Could you check a few things on this model? Use its own coordinates, in mm. A direction names the side the tool comes from. Round coordinates to 2 decimals unless told otherwise and drop trailing zeros. Loops run counter-clockwise (first coordinate to the right, second up) from the corner with the lowest first, then second, coordinate; pieces in that order, holes last. Notation, with made-up numbers: (-19.5, 88) -> (5.5, 88) arc R22 ccw to (5.5, 116) -> close; hole circle Ø8 at (49, 22.25). An arc over 180 degrees is marked (long way). Put each result on its own line as item: value. Start each with the question number.
1. Which directions (+Z, -Z, +X, -X, +Y, -Y) give clear straight access to the entire face, cutting with the end or side of a thin tool? Please do faces 1 (the flat face through (-30, 47, 14.237)), 2 (the flat face through (-16, 59, 17.767)), 3 (the cylindrical face through (-70.46, 71.27, 13.74)), 4 (the flat face through (-64, 12, 17.707)).
2. Imagine slicing it at C-C, the plane x = -95. Please give me the cut outline in (y, z).
3. Imagine slicing it at A-A, the plane z = 15.5. Please give me the cut outline in (x, y), and give its area (3 significant figures).
4. If we mould it in two halves opening along Y, with no side actions, what happens to faces 5 (the cylindrical face through (-3.177, 3.795, 13.744)), 6 (the conical face through (-18.69, 54.37, 13.46)), 7 (the flat face through (-74.272, 72, 14)), 8 (the cylindrical face through (-20.557, 52.705, 13.744))? For each: pulls with the +Y half, pulls with the -Y half, needs draft (parallel to the pull), parting line crosses it, or undercut.
5. Imagine slicing it at B-B, the plane y = -19. Please give me the cut outline in (x, z), and give its area (3 significant figures).
6. I'm going to push flat-ended pins straight in: P1, Ø2, axis at y = 24, z = 15.5, coming from the +X side; P2, Ø12, axis at x = -22.5, y = 30.5, coming from the +Z side; P3, Ø20, axis at x = -74.27, y = 0, coming from the +Z side; P4, Ø1.7, axis at x = 6.5, z = 16, coming from the -Y side. Where does each tip first touch, or does it pass through?
7. I need wall thicknesses on line 1 (Z direction, x = -11.5, y = 10.5); line 2 (Y direction, x = -69.5, z = 18.25); line 3 (Y direction, x = -32, z = 14.8). Which ranges of each line are inside material? Lowest first, please. Write a range as [from, to].
```python
from build123d import *

# Parameters (mm, degrees)
REVOLVE1_ANGLE          = 90
BOSS_EXTRUDE1_START     = -1
SKETCH2_R               = 12.5
BOSS_EXTRUDE1_DEPTH     = 1
CUT_EXTRUDE1_DEPTH      = 143.444465377
CUT_EXTRUDE1_DEPTH_BACK = 143.444465377


with BuildPart() as part:
    # Sketch1 → Revolve1 (revolve)
    with BuildSketch(Plane(origin=(0, 0, 0), x_dir=(1, 0, 0), z_dir=(0, 1, 0))):
        Polygon((-16.271625609, -17.706954757), (-19.271625609, -17.706954757), (-19.271625609, -18.706954757), (-15.861337675, -18.706954757), (-11.331165057, -14.237179487), (2.840396891, -14.237179487), (7.310172161, -18.767352105), (15.728322279, -18.767352105), (15.728322279, -17.767352105), (7.728322279, -17.767352105), (3.258547009, -13.237179487), (-11.741452991, -13.237179487), align=None)
    revolve(axis=Axis((-74.271677721, 0, 17.706954757), (0, 0, 1)), revolution_arc=REVOLVE1_ANGLE)

    # Sketch2 → Boss-Extrude1 (add)
    with BuildSketch(Plane(origin=(0, 0, 17.706954757), x_dir=(-1, 0, 0), z_dir=(0, 0, -1)).offset(BOSS_EXTRUDE1_START)):
        with BuildLine():
            Line((67.342979074, 35.326946302), (59.371742963, 52.943344025))
            ThreePointArc((59.371742963, 52.943344025), (33.582268097, 37.005103388), (20.15595474, 9.823149116))
            Line((20.15595474, 9.823149116), (39.208104561, 8.157563191))
            ThreePointArc((39.208104561, 8.157563191), (99.279307908, -25.89630152), (67.342979074, 35.326946302))
        make_face()
        with Locations((74.271677721, 0)):
            Circle(SKETCH2_R, mode=Mode.SUBTRACT)
    extrude(amount=BOSS_EXTRUDE1_DEPTH)

    # Sketch3 → Cut-Extrude1 (cut, two sides: drawn at the far end of the back side and taken through both)
    with BuildSketch(Plane(origin=(0, 0, 13.237179487), x_dir=(-1, 0, 0), z_dir=(0, 0, -1)).offset(-CUT_EXTRUDE1_DEPTH_BACK)):
        with BuildLine():
            ThreePointArc((7.421193768, 7.350328837), (3.090443615, 3.801635214), (-0.54921214, 8.056224419))
            ThreePointArc((-0.54921214, 8.056224419), (21.059515993, 53.212161728), (66.215453303, 74.820889862))
            ThreePointArc((66.215453303, 74.820889862), (70.470042507, 71.181234106), (66.921348884, 66.850483953))
            ThreePointArc((66.921348884, 66.850483953), (26.716370243, 47.555307479), (7.421193768, 7.350328837))
        make_face()
    extrude(amount=CUT_EXTRUDE1_DEPTH + CUT_EXTRUDE1_DEPTH_BACK, mode=Mode.SUBTRACT)


solid = part.part
```
Entries:
1. face 1: +Z
1. face 2: -Z, +X, +Y
1. face 3: +Z, -Z
1. face 4: -Z, -X, -Y
2. outline: (-29.43, 17.71) -> (29.43, 17.71) -> (29.43, 18.71) -> (-29.43, 18.71) -> close
3. outline: (-74.27, 60.24) arc R60.24 cw to (-14.03, 0) -> (-12.61, 0) arc R61.66 ccw to (-74.27, 61.66) -> close; (-74.27, 78.36) arc R78.36 cw to (4.09, 0) -> (5.49, 0) arc R79.76 ccw to (-74.27, 79.76) -> close
3. area: 311 mm^2
4. face 5: undercut
4. face 6: pulls with the +Y half
4. face 7: needs draft
4. face 8: undercut
5. outline: (-104.85, 17.71) -> (-43.69, 17.71) -> (-43.69, 18.71) -> (-104.85, 18.71) -> close
5. area: 61.2 mm^2
6. P1: x = 2.87
6. P2: z = 18.71
6. P3: through
6. P4: y = 0
7. line 1: [13.24, 14.24]
7. line 2: [-35.68, -11.55], [11.55, 35.68], [54.79, 58.68], [80.93, 89.87]
7. line 3: [43.9, 45.86], [65.16, 66.82]
